Read the model definition and answer for the solid it produces. Units are mm, in the model's axes. A direction names the side the tool comes from. Coordinates: 2 decimals unless noted, no trailing zeros. Write each loop counter-clockwise with the first axis right and the second up, starting at its lowest first coordinate (ties: lowest second). Pieces come first, ordered by that corner, then holes. Notation, with made-up numbers: (69, 50.5) - (117, 50.5) arc R16 ccw to (117, 75.5) - close; hole circle Ø1 at (59.25, 87). An arc over 180 degrees is marked (long way). Return JSON: item names as keys, results as strings.
```python
from build123d import *

# Parameters (mm, degrees)
SKETCH1_W           = 19.6
SKETCH1_H           = 10
BOSS_EXTRUDE1_DEPTH = 6.9
SKETCH2_W           = 0.5
SKETCH2_H           = 3.5
BOSS_EXTRUDE2_DEPTH = 4
SKETCH3_W           = 10.611233712
SKETCH3_H           = 4
BOSS_EXTRUDE3_DEPTH = 9.5
SKETCH5_R           = 1
CUT_EXTRUDE1_DEPTH  = 29.495964627


with BuildPart() as part:
    # Sketch1 → Boss-Extrude1 (new body)
    with BuildSketch(Plane(origin=(0, 0, 0), x_dir=(1, 0, 0), z_dir=(0, 1, 0))):
        with Locations((9.8, 5)):
            Rectangle(SKETCH1_W, SKETCH1_H)
    extrude(amount=BOSS_EXTRUDE1_DEPTH)

    # Sketch2 → Boss-Extrude2 (add)
    with BuildSketch(Plane.XY):
        with Locations((1.25, 3.45)):
            Rectangle(SKETCH2_W, SKETCH2_H)
        with Locations((9.05, 3.45)):
            Rectangle(SKETCH2_W, SKETCH2_H)
        with Locations((18.35, 3.45)):
            Rectangle(SKETCH2_W, SKETCH2_H)
    extrude(amount=BOSS_EXTRUDE2_DEPTH)

    # Sketch3 → Boss-Extrude3 (add)
    with BuildSketch(Plane(origin=(0, 0, -10), x_dir=(-1, 0, 0), z_dir=(0, 0, -1))):
        with Locations((-14.294383144, 3.45)):
            Rectangle(SKETCH3_W, SKETCH3_H)
    extrude(amount=BOSS_EXTRUDE3_DEPTH)

    # Sketch5 → Cut-Extrude1 (cut, through all)
    with BuildSketch(Plane(origin=(0, 6.9, 0), x_dir=(1, 0, 0), z_dir=(0, 1, 0))):
        with Locations(Location((5.05, 2.5, 0), (0, 0, 270))):
            Circle(SKETCH5_R)
        with Locations(Location((14.55, 2.5, 0), (0, 0, 270))):
            Circle(SKETCH5_R)
    extrude(amount=-CUT_EXTRUDE1_DEPTH, mode=Mode.SUBTRACT)


solid = part.part
```
(1) Straight lines are drawn through the part: line 1 (X direction, y = 2.5, z = -2.5); line 2 (Z direction, x = 10, y = 5.5); line 3 (Y direction, x = 16.25, z = -16.25). For each, find the intervals that lie inside material, in ascending order. Write a range as from..to.
Answer:
{"line 1": "0..4.05, 6.05..13.55, 15.55..19.6", "line 2": "-10..0", "line 3": "1.45..5.45"}
(2) Which of the six approach directions +Z, -Z, +X, -X, +Y, -Y give full straight-line access (tool end or side, diameter ignored) to faces 4 (the face through (14, 5.45, -15)), 5 (the face through (9.3, 3, 2)), 6 (the face through (14, 1.45, -15))?
Answer:
{"face 4": "-Z, +X, -X, +Y", "face 5": "+Z, +Y, -Y", "face 6": "-Z, +X, -X, -Y"}
(3) Flat-ended cylindrical pins translate along their axes: P1, Ø3, axis at y = 3, z = 2, coming from the +X side; P2, Ø2, axis at y = 2.5, z = -4, coming from the -X side; P3, Ø0.6, axis at x = 18.5, z = 2, coming from the -Y side; P4, Ø2, axis at x = 12, z = -17, coming from the +Y side. Find the tip coordinate at first contact, or state that the pin passes through.
Answer:
{"P1": "x = 18.6", "P2": "x = 0", "P3": "y = 1.7", "P4": "y = 5.45"}
(4) A cutting plane is placed at A-A (z = -2.5). Determine the outline of the cut face in (x, y).
Answer:
{"outline": "(0, 0) - (4.05, 0) - (4.05, 6.9) - (0, 6.9) - close; (6.05, 0) - (13.55, 0) - (13.55, 6.9) - (6.05, 6.9) - close; (15.55, 0) - (19.6, 0) - (19.6, 6.9) - (15.55, 6.9) - close"}
(5) A cutting plane is placed at B-B (x = 5.05). Determine the outline of the cut face in (y, z).
Answer:
{"outline": "(0, -10) - (6.9, -10) - (6.9, -3.5) - (0, -3.5) - close; (0, -1.5) - (6.9, -1.5) - (6.9, 0) - (0, 0) - close"}
(6) A cutting plane is placed at D-D (x = 12). Determine the outline of the cut face in (y, z), and give its area (3 significant figures).
Answer:
{"outline": "(0, -10) - (1.45, -10) - (1.45, -19.5) - (5.45, -19.5) - (5.45, -10) - (6.9, -10) - (6.9, 0) - (0, 0) - close", "area": "107 mm²"}
(7) A cutting plane is placed at C-C (y = 4). Determine the outline of the cut face in (x, z).
Answer:
{"outline": "(0, -10) - (8.99, -10) - (8.99, -19.5) - (19.6, -19.5) - (19.6, 0) - (18.6, 0) - (18.6, 4) - (18.1, 4) - (18.1, 0) - (9.3, 0) - (9.3, 4) - (8.8, 4) - (8.8, 0) - (1.5, 0) - (1.5, 4) - (1, 4) - (1, 0) - (0, 0) - close; hole circle Ø2 at (5.05, -2.5); hole circle Ø2 at (14.55, -2.5)"}
(8) Determine the mould class of faces 1 (the face through (0, 3, -5)), 2 (the face through (7, 3, -10)), 3 (the face through (18.1, 3, 2)) for opening direction X: +X half, -X half, draft (parallel to the pull), parting line (faces both ways), or undercut.
Answer:
{"face 1": "-X half", "face 2": "draft", "face 3": "undercut"}
